from build123d import *

# Parameters (mm, degrees)
F0_R     = 19.05
F1_DEPTH = 9.525
F2_SIZE  = 1.27


# Not quite as in the source:
# - a feature names something its author has since deleted; it is built from what else it names


with BuildPart() as f1:
    # F0 (on Front) → F1 (new body, symmetric)
    with BuildSketch(Plane.XZ):
        with BuildLine():
            Line((-101.4069377299, 8.9171452969), (-12.5069377299, -29.1828547031))
            ThreePointArc((-12.5069377299, -29.1828547031), (0, -31.75), (12.5069377299, -29.1828547031))
            Line((12.5069377299, -29.1828547031), (101.4069377299, 8.9171452969))
            ThreePointArc((101.4069377299, 8.9171452969), (117.9736119422, 50.8588239518), (75.8902439024, 67.062195122))
            ThreePointArc((75.8902439024, 67.062195122), (0, 50.8), (-75.8902439024, 67.062195122))
            ThreePointArc((-75.8902439024, 67.062195122), (-117.9736119422, 50.8588239518), (-101.4069377299, 8.9171452969))
        make_face()
        Circle(F0_R, mode=Mode.SUBTRACT)
        with Locations((-88.9, 38.1)):
            Circle(F0_R, mode=Mode.SUBTRACT)
        with Locations((88.9, 38.1)):
            Circle(F0_R, mode=Mode.SUBTRACT)
    extrude(amount=F1_DEPTH, both=True)

    # F2
    f2_edges = [f1.edges().sort_by_distance(p)[0] for p in [
        (-117.973612, -9.525, 50.858824),
        (-56.956938, -9.525, -10.132855),
        (0, -9.525, -31.75),
        (56.956938, -9.525, -10.132855),
        (117.973612, -9.525, 50.858824),
        (0, -9.525, 50.8),
        (-56.956938, 9.525, -10.132855),
        (0, 9.525, -31.75),
        (56.956938, 9.525, -10.132855),
        (117.973612, 9.525, 50.858824),
        (0, 9.525, 50.8),
        (-117.973612, 9.525, 50.858824),
        (-19.05, 9.525, 0),
        (-107.95, 9.525, 38.1),
        (69.85, 9.525, 38.1),
        (-19.05, -9.525, 0),
        (-107.95, -9.525, 38.1),
        (69.85, -9.525, 38.1),
    ]]
    chamfer(f2_edges, length=F2_SIZE)


solid = f1.part
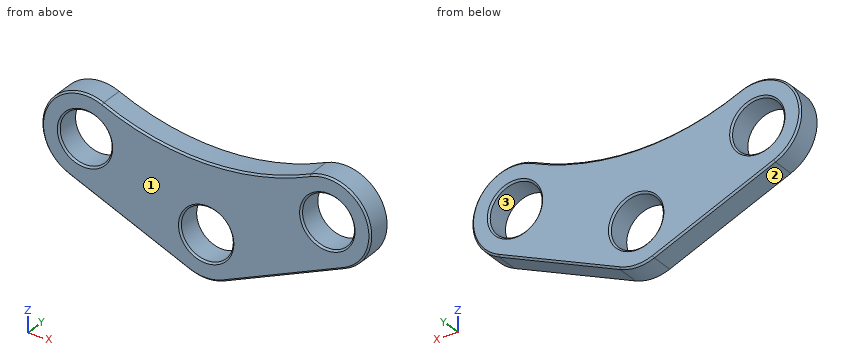
Source: CAD feature listing. Evaluate the final solid. Frame: model axes, mm. Face numbers are marked on the shaded views. Round coordinates to 2 decimals unless told otherwise and drop trailing zeros. Order: outer loops, then holes, each group sorted by start corner. A loop starts at its lowest first (then second) coordinate and runs counter-clockwise, first axis right, second up. Notation, with made-up numbers: (-15, 5) - (-3, 5) arc R18 cw to (-3, 27) - close; hole circle Ø4 at (52, -24.5). An arc over 180 degrees is marked (long way). Use a Markdown table: item, result. Add a question column.
1. Section query C-C (x = 88.9). Return the cut outline in (y, z) (3 decimals), then the cut area to 3 significant figures.
2. Mould query, pull axis X, two halves, no side actions, for the marked faces 1, 2 and 3. Classes: +X half, -X half, draft (parallel to the pull), parting line (faces both ways), or undercut.
3. Section query A-A (z = 38.1). Return the cut outline in (x, y) (3 decimals), then the cut area to 3 significant figures.
4. Section query B-B (y = -4.5). Return the cut outline in (x, z), then the cut area to 3 significant figures.
5. Line query: probe 1 along X at (y, z) = (-1, 37.5); probe 2 along X at (y, z) = (7, 25.5); probe 3 along Z at (x, y) = (-13.5, 8). Output: solid intervals per line, ascending.
6. Section query D-D (z = 0). Return the cut outline in (x, y) (3 decimals), then the cut area to 3 significant figures.
7. First-contact query: pin 1 (3 mm diameter, centred on x = 34, y = -2.5, fed in from -Z); pin 2 (10 mm diameter, centred on x = -62.5, y = -6.5, fed in from +Z); pin 3 (1 mm diameter, centred on x = -54.5, y = 0, fed in from +Z). Flat tips, straight axial feed; report the tip coordinate or a pass-through.
Derived:
| question | item | result |
|---|---|---|
| 1 | outline | (-9.525, 4.939) - (-8.255, 3.557) - (8.255, 3.557) - (9.525, 4.939) - (9.525, 17.78) - (8.255, 19.05) - (-8.255, 19.05) - (-9.525, 17.78) - close; (-9.525, 58.42) - (-8.255, 57.15) - (8.255, 57.15) - (9.525, 58.42) - (9.525, 68.58) - (8.255, 69.85) - (-8.255, 69.85) - (-9.525, 68.58) - close |
| 1 | area | 530 mm2 |
| 2 | face 1 | draft |
| 2 | face 2 | -X half |
| 2 | face 3 | undercut |
| 3 | outline | (-120.65, -8.255) - (-119.38, -9.525) - (-109.22, -9.525) - (-107.95, -8.255) - (-107.95, 8.255) - (-109.22, 9.525) - (-119.38, 9.525) - (-120.65, 8.255) - close; (-69.85, -8.255) - (-68.58, -9.525) - (68.58, -9.525) - (69.85, -8.255) - (69.85, 8.255) - (68.58, 9.525) - (-68.58, 9.525) - (-69.85, 8.255) - close; (107.95, -8.255) - (109.22, -9.525) - (119.38, -9.525) - (120.65, -8.255) - (120.65, 8.255) - (119.38, 9.525) - (109.22, 9.525) - (107.95, 8.255) - close |
| 3 | area | 3,140 mm2 |
| 4 | outline | (-101.41, 8.92) - (-12.51, -29.18) arc R31.75 ccw to (12.51, -29.18) - (101.41, 8.92) arc R31.75 ccw (long way) to (75.89, 67.06) arc R185.21 cw to (-75.89, 67.06) arc R31.75 ccw (long way) to start; hole circle Ø38.1 at (-88.9, 38.1); hole circle Ø38.1 at (0, 0); hole circle Ø38.1 at (88.9, 38.1) |
| 4 | area | 12,800 mm2 |
| 5 | probe 1 | -120.64 to -107.94, -69.86 to 69.86, 107.94 to 120.64 |
| 5 | probe 2 | -118.04 to -103.19, -74.61 to 74.61, 103.19 to 118.04 |
| 5 | probe 3 | -28.76 to -13.44, 13.44 to 51.29 |
| 6 | outline | (-80.6, -8.255) - (-77.376, -9.525) - (-20.32, -9.525) - (-19.05, -8.255) - (-19.05, 8.255) - (-20.32, 9.525) - (-77.376, 9.525) - (-80.6, 8.255) - close; (19.05, -8.255) - (20.32, -9.525) - (77.376, -9.525) - (80.6, -8.255) - (80.6, 8.255) - (77.376, 9.525) - (20.32, 9.525) - (19.05, 8.255) - close |
| 6 | area | 2,330 mm2 |
| 7 | pin 1 | z = -20.61 |
| 7 | pin 2 | z = 63.54 |
| 7 | pin 3 | z = 59.15 |
